Can you work these out from the model? Positions are in its coordinate system, mm. A direction names the side the tool comes from. Round coordinates to 2 decimals unless told otherwise and drop trailing zeros. Write each loop counter-clockwise with the first axis right and the second up, starting at its lowest first coordinate (ties: lowest second). Pieces come first, ordered by that corner, then holes.
Q1. We'd pull the mould along Z, two halves only. Please class faces 1 (the cylindrical face through (0.044, 4.444, -27.101)), 2 (the cylindrical face through (-3.27, -0.02, -49.9)), 3 (the flat face through (1.588, 3, -27)): +Z half, -Z half, draft (parallel to the pull), parting line (faces both ways), or undercut.
Q2. I'm going to push flat-ended pins straight in: pin 1 Ø2 at (x, z) = (-1, -44.5) entering from +Y; pin 2 Ø1.3 at (y, z) = (-0.5, -22.5) entering from +X (3 decimals); pin 3 Ø1.3 at (y, z) = (3, -24) entering from -X. Where does each tip first touch, or does it pass through?
Q3. If we section it at D-D (y = 2.25): Please give me the cut outline in (x, z), plus the area to 3 significant figures.
Q4. If we section it at A-A (y = -0.4): Please give me the cut outline in (x, z) (1 decimal), plus the area to 3 significant figures.
Q5. Please list where these lines run through material, in increasing order: line 1 along Z through (x, y) = (-0.5, 0.6); line 2 along Z through (x, y) = (1, 0.75); line 3 along X through (y, z) = (-0.5, -48.5) (3 decimals).
Q6. If we section it at C-C (x = 0): Please give me the cut outline in (y, z).
Q7. If we section it at B-B (z = 0): Please give me the cut outline in (x, y), plus the area to 3 significant figures.
Q8. For faces 4 (the cylindrical face through (3.28, -0.02, -49.92)), 5 (the flat face through (-1.588, 3, -27)), 6 (the flat face through (-3.175, 0, -26)), 7 (the flat face through (0, -1.27, -27)), which set-ups out of +Z, -Z, +X, -X, +Y, -Y let a thin tool reach every point of the face, with its end or its side?
from build123d import *

# Parameters (mm, degrees)
SKETCH1_R           = 1.5875
BOSS_EXTRUDE1_DEPTH = 1.27
BOSS_EXTRUDE2_DEPTH = 1.5875
FILLET1_R           = 1.524


with BuildPart() as part:
    # Sketch1 → Boss-Extrude1 (new body, symmetric)
    with BuildSketch(Plane(origin=(0, 0, 0), x_dir=(1, 0, 0), z_dir=(0, 1, 0))):
        with BuildLine():
            Line((-3.175, 3.549757914), (-3.175, 49.993442086))
            ThreePointArc((-3.175, 49.993442086), (0, 58.3057), (3.175, 49.993442086))
            Line((3.175, 49.993442086), (3.175, 3.549757914))
            ThreePointArc((3.175, 3.549757914), (0, -4.7625), (-3.175, 3.549757914))
        make_face()
        Circle(SKETCH1_R, mode=Mode.SUBTRACT)
        with Locations((0, 53.5432)):
            Circle(SKETCH1_R, mode=Mode.SUBTRACT)
    extrude(amount=BOSS_EXTRUDE1_DEPTH, both=True)

    # Sketch2 → Cut-Revolve1 (revolve, cut)
    with BuildSketch(Plane(origin=(0, 0, 0), x_dir=(0, 0, -1), z_dir=(1, 0, 0))):
        with BuildLine():
            Line((0, -2.54), (0, 2.54))
            ThreePointArc((0, 2.54), (2.54, 0), (0, -2.54))
        make_face()
    revolve(axis=Axis((0, -2.54, 0), (0, 1, 0)), mode=Mode.SUBTRACT)

    # Sketch3 → Cut-Revolve2 (revolve, cut)
    with BuildSketch(Plane(origin=(0, 0, 0), x_dir=(0, 0, -1), z_dir=(1, 0, 0))):
        with BuildLine():
            Line((53.574492193, -2.54), (53.574492193, 2.54))
            ThreePointArc((53.574492193, 2.54), (51.034492193, 0), (53.574492193, -2.54))
        make_face()
    revolve(axis=Axis((0, 8.508702539, -53.574492193), (0, -1, 0)), mode=Mode.SUBTRACT)

    # Sketch5 → Boss-Extrude2 (add, symmetric)
    with BuildSketch(Plane(origin=(0, 0, 0), x_dir=(0, 0, -1), z_dir=(1, 0, 0))):
        with BuildLine():
            Line((3.549757914, 1.27), (49.993442086, 1.27))
            ThreePointArc((49.993442086, 1.27), (26.7716, 4.445), (3.549757914, 1.27))
        make_face()
    extrude(amount=BOSS_EXTRUDE2_DEPTH, both=True)

    # Fillet1
    fillet1_edges = [part.edges().sort_by_distance(p)[0] for p in [
        (-1.5875, 1.27, -26.7716),
        (1.5875, 1.27, -26.7716),
        (-3.175, 0, -3.549757914),
        (-3.175, 0, -49.993442086),
        (3.175, 0, -49.993442086),
        (3.175, 0, -3.549757914),
    ]]
    fillet(fillet1_edges, radius=FILLET1_R)


solid = part.part
A:
1. face 1: parting line
1. face 2: undercut
1. face 3: draft
2. pin 1: stops at y = 2.81
2. pin 2: stops at x = 3.175
2. pin 3: stops at x = -1.65
3. outline: (-1.69, -46.14) - (1.69, -46.14) - (1.69, -7.41) - (-1.69, -7.41) - close
3. area: 131 mm2
4. outline: (-3.6, -50.4) arc R4.8 ccw (long way) to (3.6, -50.4) arc R1.5 cw to (3.2, -49.4) - (3.2, -4.2) arc R1.5 cw to (3.6, -3.2) arc R4.8 ccw (long way) to (-3.6, -3.2) arc R1.5 cw to (-3.2, -4.2) - (-3.2, -49.4) arc R1.5 cw to start; hole circle Ø5 at (0, -53.6); hole circle Ø5 at (0, 0)
4. area: 388 mm2
5. line 1: z = -58.28 to -55.99, -51.16 to -2.42, 2.42 to 4.74
5. line 2: z = -58.2 to -55.79, -51.36 to -2.21, 2.21 to 4.66
5. line 3: x = -3.175 to 3.175
6. outline: (-1.27, -58.31) - (1.27, -58.31) - (1.27, -55.77) arc R2.54 cw to (-1.27, -55.77) - close; (-1.27, -51.37) arc R2.54 cw to (1.27, -51.37) - (1.27, -49.99) arc R86.51 ccw to (1.27, -3.55) - (1.27, -2.2) arc R2.54 cw to (-1.27, -2.2) - close; (-1.27, 2.2) arc R2.54 cw to (1.27, 2.2) - (1.27, 4.76) - (-1.27, 4.76) - close
7. outline: (-4.76, -1.27) - (-2.2, -1.27) arc R2.54 cw to (-2.2, 1.27) - (-4.76, 1.27) - close; (2.2, -1.27) - (4.76, -1.27) - (4.76, 1.27) - (2.2, 1.27) arc R2.54 cw to start
7. area: 11.9 mm2
8. face 4: +X, +Y, -Y
8. face 5: +Z, -Z, -X, +Y
8. face 6: -X, +Y, -Y
8. face 7: +Z, -Z, +X, -X, -Y
